from build123d import *

# Parameters (mm, degrees)
CYLINDER529_R     = 1.5
CYLINDER529_DEPTH = 100
CYLINDER528_R     = 1.5
CYLINDER528_DEPTH = 100
CYLINDER367_R     = 3
CYLINDER367_DEPTH = 4
CYLINDER365_R     = 1.5
CYLINDER365_DEPTH = 50
CYLINDER360_R     = 3
CYLINDER360_DEPTH = 4
CYLINDER359_R     = 3
CYLINDER359_DEPTH = 4
CYLINDER356_R     = 3
CYLINDER356_DEPTH = 4
CYLINDER353_R     = 3
CYLINDER353_DEPTH = 4
CYLINDER350_R     = 1.5
CYLINDER350_DEPTH = 50
CYLINDER349_R     = 1.5
CYLINDER349_DEPTH = 50
CYLINDER347_R     = 1.5
CYLINDER347_DEPTH = 50
CYLINDER348_R     = 1.5
CYLINDER348_DEPTH = 50
CYLINDER346_R     = 1.5
CYLINDER346_DEPTH = 100
CYLINDER345_R     = 1.5
CYLINDER345_DEPTH = 100
CYLINDER287_R     = 59
CYLINDER287_DEPTH = 2


with BuildPart() as obj1:
    # Cylinder529 → Cylinder529 (new body)
    with BuildSketch(Plane(origin=(39, -21, 0), x_dir=(1, 0, 0), z_dir=(0, 0, 1))):
        Circle(CYLINDER529_R)
    extrude(amount=CYLINDER529_DEPTH)


with BuildPart() as compound:
    # Cylinder528 → Cylinder528 (new body)
    with BuildSketch(Plane(origin=(-39, -21, 0), x_dir=(1, 0, 0), z_dir=(0, 0, 1))):
        Circle(CYLINDER528_R)
    extrude(amount=CYLINDER528_DEPTH)

    # Compound: union obj1
    add(obj1.part)


with BuildPart() as obj2:
    # Cylinder367 → Cylinder367 (new body)
    with BuildSketch(Plane(origin=(0, -50, 9), x_dir=(1, 0, 0), z_dir=(0, 0, 1))):
        Circle(CYLINDER367_R)
    extrude(amount=CYLINDER367_DEPTH)


with BuildPart() as obj3:
    # Cylinder365 → Cylinder365 (new body)
    with BuildSketch(Plane(origin=(0, 50, 0), x_dir=(1, 0, 0), z_dir=(0, 0, 1))):
        Circle(CYLINDER365_R)
    extrude(amount=CYLINDER365_DEPTH)


with BuildPart() as obj4:
    # Cylinder360 → Cylinder360 (new body)
    with BuildSketch(Plane(origin=(-34, -36, 0), x_dir=(1, 0, 0), z_dir=(0, 0, 1))):
        Circle(CYLINDER360_R)
    extrude(amount=CYLINDER360_DEPTH)


with BuildPart() as compound305:
    # Cylinder359 → Cylinder359 (new body)
    with BuildSketch(Plane(origin=(34, -36, 0), x_dir=(1, 0, 0), z_dir=(0, 0, 1))):
        Circle(CYLINDER359_R)
    extrude(amount=CYLINDER359_DEPTH)

    # Compound305: union obj4
    add(obj4.part)


with BuildPart() as compound305_1:
    # Compound305 placement: moved
    add(compound305.part.moved(Location((0, 0, 9))))


with BuildPart() as obj5:
    # Cylinder356 → Cylinder356 (new body)
    with BuildSketch(Plane(origin=(24, 18, 0), x_dir=(1, 0, 0), z_dir=(0, 0, 1))):
        Circle(CYLINDER356_R)
    extrude(amount=CYLINDER356_DEPTH)


with BuildPart() as compound304:
    # Cylinder353 → Cylinder353 (new body)
    with BuildSketch(Plane(origin=(-24, 18, 0), x_dir=(1, 0, 0), z_dir=(0, 0, 1))):
        Circle(CYLINDER353_R)
    extrude(amount=CYLINDER353_DEPTH)

    # Compound304: union obj5
    add(obj5.part)


with BuildPart() as compound304_1:
    # Compound304 placement: moved
    add(compound304.part.moved(Location((0, 0, 10))))


with BuildPart() as obj6:
    # Cylinder350 → Cylinder350 (new body)
    with BuildSketch(Plane(origin=(-34, 36, 0), x_dir=(1, 0, 0), z_dir=(0, 0, 1))):
        Circle(CYLINDER350_R)
    extrude(amount=CYLINDER350_DEPTH)


with BuildPart() as obj7:
    # Cylinder349 → Cylinder349 (new body)
    with BuildSketch(Plane(origin=(34, 36, 0), x_dir=(1, 0, 0), z_dir=(0, 0, 1))):
        Circle(CYLINDER349_R)
    extrude(amount=CYLINDER349_DEPTH)


with BuildPart() as obj8:
    # Cylinder347 → Cylinder347 (new body)
    with BuildSketch(Plane(origin=(51, 6, 0), x_dir=(1, 0, 0), z_dir=(0, 0, 1))):
        Circle(CYLINDER347_R)
    extrude(amount=CYLINDER347_DEPTH)


with BuildPart() as obj9:
    # Cylinder348 → Cylinder348 (new body)
    with BuildSketch(Plane(origin=(-51, 6, 0), x_dir=(1, 0, 0), z_dir=(0, 0, 1))):
        Circle(CYLINDER348_R)
    extrude(amount=CYLINDER348_DEPTH)


with BuildPart() as obj10:
    # Cylinder346 → Cylinder346 (new body)
    with BuildSketch(Plane(origin=(51, -12, 0), x_dir=(1, 0, 0), z_dir=(0, 0, 1))):
        Circle(CYLINDER346_R)
    extrude(amount=CYLINDER346_DEPTH)


with BuildPart() as compound302:
    # Cylinder345 → Cylinder345 (new body)
    with BuildSketch(Plane(origin=(-51, -12, 0), x_dir=(1, 0, 0), z_dir=(0, 0, 1))):
        Circle(CYLINDER345_R)
    extrude(amount=CYLINDER345_DEPTH)

    # Compound302: union obj6, obj7, obj8, obj9, obj10
    add(obj6.part)
    add(obj7.part)
    add(obj8.part)
    add(obj9.part)
    add(obj10.part)


with BuildPart() as cut160:
    # Cylinder287 → Cylinder287 (new body)
    with BuildSketch(Plane.XY.offset(10)):
        Circle(CYLINDER287_R)
    extrude(amount=CYLINDER287_DEPTH)

    # Cut148: cut Compound302
    add(compound302.part, mode=Mode.SUBTRACT)

    # Cut149: cut Compound304
    add(compound304_1.part, mode=Mode.SUBTRACT)

    # Cut150: cut Compound305
    add(compound305_1.part, mode=Mode.SUBTRACT)

    # Cut155: cut obj3
    add(obj3.part, mode=Mode.SUBTRACT)

    # Cut157: cut obj2
    add(obj2.part, mode=Mode.SUBTRACT)

    # Cut160: cut Compound
    add(compound.part, mode=Mode.SUBTRACT)


solid = cut160.part
Design review of the part built by this model. Coordinates are the model's own, in mm. Coordinates: 2 decimals unless noted, no trailing zeros. Order: outer loops, then holes, each group sorted by start corner. A loop starts at its lowest first (then second) coordinate and runs counter-clockwise, first axis right, second up. Notation, with made-up numbers: M 70.5,-0.5 L 88.5,-0.5 A34 cw 88.5,32.5 Z; hole C -12,68.25 d5. An arc over 180 degrees is marked long. Use a Markdown table: item, result.
(1) Add section D-D (y = -12). Give the boundary of the cut face in (x, z), then the cut area to 3 significant figures.
Worked answers:
| item | result |
|---|---|
| outline | M -57.77,10 L -52.5,10 L -52.5,12 L -57.77,12 Z; M -49.5,10 L 49.5,10 L 49.5,12 L -49.5,12 Z; M 52.5,10 L 57.77,10 L 57.77,12 L 52.5,12 Z |
| area | 219 mm2 |
(2) Add section C-C (y = 50). Give the boundary of the cut face in (x, z), then the cut area to 3 significant figures.
Worked answers:
| item | result |
|---|---|
| outline | M -31.32,10 L -1.5,10 L -1.5,12 L -31.32,12 Z; M 1.5,10 L 31.32,10 L 31.32,12 L 1.5,12 Z |
| area | 119 mm2 |
(3) Draft analysis for pull direction X (two halves, no side actions). For faces 1 (the cylindrical face through (49.5, 6.07, 10.99)), 2 (the flat face through (-1, 1, 10)), 3 (the cylindrical face through (56.275, 17.722, 10.986)), 4 (the cylindrical face through (49.5, -11.93, 10.99)), state which applies: released by +X, released by -X, zero draft, split by the parting line, or undercut.
Worked answers:
| item | result |
|---|---|
| face 1 | undercut |
| face 2 | zero draft |
| face 3 | split by the parting line |
| face 4 | undercut |
(4) Wall thickness on probe 1 along X at (y, z) = (36, 11.5); probe 2 along Y at (x, z) = (51, 11.35); probe 3 along Y at (x, z) = (50, 10.5): over which ranges is each line inside the solid? List them lowest first.
Worked answers:
| item | result |
|---|---|
| probe 1 | x = -46.74 to -35.5, -32.5 to 32.5, 35.5 to 46.74 |
| probe 2 | y = -29.66 to -13.5, -10.5 to 4.5, 7.5 to 29.66 |
| probe 3 | y = -31.32 to -13.12, -10.88 to 4.88, 7.12 to 31.32 |
(5) Add section A-A (z = 11.6). Count the separate pieces of the cut face and the enclosed holes in it, then the cut area to 3 significant figures.
Worked answers:
| item | result |
|---|---|
| separate pieces | 1 |
| enclosed holes | 14 |
| area | 10,700 mm2 |
(6) Add section B-B (x = 0). Give the boundary of the cut face in (y, z), then the cut area to 3 significant figures.
Worked answers:
| item | result |
|---|---|
| outline | M -59,10 L -53,10 L -53,12 L -59,12 Z; M -47,10 L 48.5,10 L 48.5,12 L -47,12 Z; M 51.5,10 L 59,10 L 59,12 L 51.5,12 Z |
| area | 218 mm2 |
